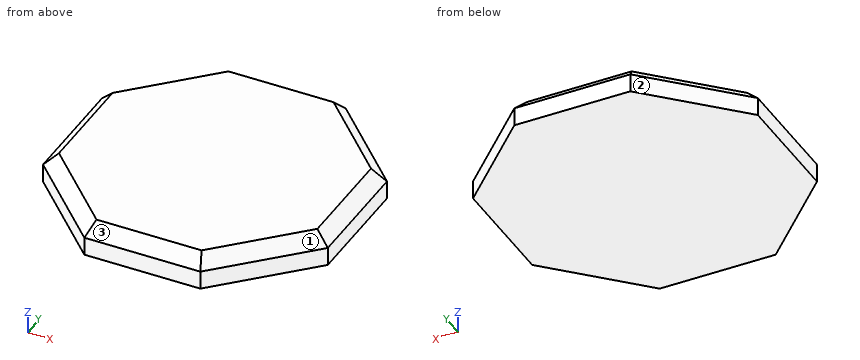
```python
from build123d import *

# Parameters (mm, degrees)
F0_W      = 171.45
F0_H      = 171.45
F1_DEPTH  = 19.05
F3_DEPTH  = 127
F2_W      = 12.7
F2_H      = 17.1814748066
F4_DEPTH  = 203.2
F5_SIZE   = 5.08
F6_DEPTH  = 177.8
F7_SIZE   = 5.08
F8_DEPTH  = 177.8
F9_SIZE   = 5.08
F2_H_2    = 15.875
F10_DEPTH = 152.4
F11_SIZE  = 5.08
F12_SIZE  = 50.8
F13_SIZE  = 7.9375
F15_R     = 19.8103080262
F16_DEPTH = 355.6
F17_SIZE  = 5.08
F18_DEPTH = 25.4


with BuildPart() as f1:
    # F0 (on Top) → F1 (new body)
    with BuildSketch(Plane.XY):
        Rectangle(F0_W, F0_H)
    extrude(amount=F1_DEPTH)

    # F12
    f12_edges = [f1.edges().sort_by_distance(p)[0] for p in [
        (85.725, 85.725, 9.525),
        (-85.725, 85.725, 9.525),
        (85.725, -85.725, 9.525),
        (-85.725, -85.725, 9.525),
    ]]
    chamfer(f12_edges, length=F12_SIZE)

    # F13
    f13_edges = [f1.edges().sort_by_distance(p)[0] for p in [
        (-60.325, -60.325, 19.05),
        (0, -85.725, 19.05),
        (60.325, -60.325, 19.05),
        (85.725, 0, 19.05),
        (60.325, 60.325, 19.05),
        (0, 85.725, 19.05),
        (-60.325, 60.325, 19.05),
        (-85.725, 0, 19.05),
    ]]
    chamfer(f13_edges, length=F13_SIZE)


with BuildPart() as f3:
    # F2 (on face) → F3 (new body)
    with BuildSketch(Plane.XY.offset(19.05)):
        Polygon((-8.0955186849, -20.6375), (7.9502, -20.6375), (20.6375, -9.2439748066), (20.6375, 7.9375), (7.9502, 20.6375), (-7.8052744357, 20.6375), (-20.6375, 7.9375), (-20.6375, -7.9375), align=None)
    extrude(amount=F3_DEPTH)


with BuildPart() as f4:
    # F2 (on face) → F4 (new body)
    with BuildSketch(Plane.XY.offset(19.05)):
        with Locations((26.9875, -0.6532374033)):
            Rectangle(F2_W, F2_H)
    extrude(amount=F4_DEPTH)

    # F5
    f5_edges = [f4.edges().sort_by_distance(p)[0] for p in [
        (33.3375, -0.653237, 222.25),
    ]]
    chamfer(f5_edges, length=F5_SIZE)


with BuildPart() as f6:
    # F2 (on face) → F6 (new body)
    with BuildSketch(Plane.XY.offset(19.05)):
        Polygon((-8.1848246077, -33.3375), (7.9502, -33.3375), (7.9502, -20.6375), (-8.0955186849, -20.6375), align=None)
    extrude(amount=F6_DEPTH)

    # F7
    f7_edges = [f6.edges().sort_by_distance(p)[0] for p in [
        (-0.117312, -33.3375, 196.85),
    ]]
    chamfer(f7_edges, length=F7_SIZE)


with BuildPart() as f8:
    # F2 (on face) → F8 (new body)
    with BuildSketch(Plane.XY.offset(19.05)):
        Polygon((-7.8052744357, 20.6375), (7.9502, 20.6375), (7.9502, 33.3375), (-7.7159685129, 33.3375), align=None)
    extrude(amount=F8_DEPTH)

    # F9
    f9_edges = [f8.edges().sort_by_distance(p)[0] for p in [
        (0.117116, 33.3375, 196.85),
    ]]
    chamfer(f9_edges, length=F9_SIZE)


with BuildPart() as f10:
    # F2 (on face) → F10 (new body)
    with BuildSketch(Plane.XY.offset(19.05)):
        with Locations((-26.9875, 0)):
            Rectangle(F2_W, F2_H_2)
    extrude(amount=F10_DEPTH)

    # F11
    f11_edges = [f10.edges().sort_by_distance(p)[0] for p in [
        (-33.3375, 0, 171.45),
    ]]
    chamfer(f11_edges, length=F11_SIZE)


with BuildPart() as f16:
    # F15 (on face) → F16 (new body)
    with BuildSketch(Plane.XY.offset(146.05)):
        Circle(F15_R)
    extrude(amount=F16_DEPTH)

    # F17
    f17_edges = [f16.edges().sort_by_distance(p)[0] for p in [
        (-19.810308, 0, 501.65),
    ]]
    chamfer(f17_edges, length=F17_SIZE)


with BuildPart() as f18:
    # F14 (on face) → F18 (new body)
    with BuildSketch(Plane.XY.offset(146.05)):
        with BuildLine():
            Line((20.6375, -0.9718922405), (20.6375, 0.9718922405))
            ThreePointArc((20.6375, 0.9718922405), (19.6667538049, 6.3300691588), (17.3298010521, 11.2485099579))
            Line((17.3298010521, 11.2485099579), (11.2658427939, 17.3185382443))
            ThreePointArc((11.2658427939, 17.3185382443), (6.3399066616, 19.6635847266), (0.9718922405, 20.6375))
            Line((0.9718922405, 20.6375), (-0.9718922405, 20.6375))
            ThreePointArc((-0.9718922405, 20.6375), (-6.1694748401, 19.7177220027), (-10.9643715831, 17.5109547588))
            Line((-10.9643715831, 17.5109547588), (-17.3964546014, 11.1451490829))
            ThreePointArc((-17.3964546014, 11.1451490829), (-19.685507724, 6.2715043193), (-20.6375, 0.9718922405))
            Line((-20.6375, 0.9718922405), (-20.6375, -0.9718922405))
            ThreePointArc((-20.6375, -0.9718922405), (-19.6458745255, -6.3945754282), (-17.2555997462, -11.3620094251))
            Line((-17.2555997462, -11.3620094251), (-11.5771558663, -17.1119970437))
            ThreePointArc((-11.5771558663, -17.1119970437), (-6.5174339176, -19.6054593393), (-0.9718922405, -20.6375))
            Line((-0.9718922405, -20.6375), (0.9718922405, -20.6375))
            ThreePointArc((0.9718922405, -20.6375), (14.6090893073, -14.6090893073), (20.6375, -0.9718922405))
        make_face()
    extrude(amount=F18_DEPTH)


solid = f1.part
```
CAD build for the part. Positions are in the model's coordinates, mm. Face numbers are marked on the shaded views. Round coordinates to 2 decimals unless told otherwise and drop trailing zeros. Write each loop counter-clockwise with the first axis right and the second up, starting at its lowest first coordinate (ties: lowest second). Pieces come first, ordered by that corner, then holes. Notation, with made-up numbers: (77.25, 55.5) - (87.25, 55.5) arc R26 cw to (87.25, 92.5) - close; hole circle Ø8 at (24, 22). An arc over 180 degrees is marked (long way). Write item = value, one per line. Start each with the question number.
Q1. Mould opens along X. For the marked faces 1, 2 and 3 say: pulls with the +X half, pulls with the -X half, needs draft (parallel to the pull), parting line crosses it, or undercut.
Q2. Drop flat-ended pins along their axis: pin 1 (6 mm diameter, centred on x = -62.5, y = -16.5, fed in from -Z); pin 2 (3 mm diameter, centred on y = -20.5, z = 17, fed in from +X); pin 3 (2 mm diameter, centred on x = 58.5, z = 14, fed in from -Y); pin 4 (1 mm diameter, centred on x = 20.5, z = 13.5, fed in from -Y). Give the stop position or say it passes through.
Q3. Probe L1, parallel to Y at x = -76.5, z = 12.75; L2, parallel to X at y = -54, z = 3.75; L3, parallel to Z at x = -70, y = 44.5. List the from-to ranges inside material, lowest first. Write a range as from..to.
Q4. Band-saw the part on D-D (z = 16). Give the cut face in (x, y).
Q5. Band-saw the part on B-B (z = 5.5). Give the cut face in (x, y) (3 decimals).
Answers below:
q1.face_1 = pulls with the +X half
q1.face_2 = pulls with the -X half
q1.face_3 = needs draft
q2.pin_1 = 0
q2.pin_2 = 81.34
q2.pin_3 = -59.8
q2.pin_4 = -83.84
q3.L1 = -41.83..41.83
q3.L2 = -66.65..66.65
q3.L3 = 0..15.46
q4.outline = (-80.84, -32.9) - (-32.9, -80.84) - (32.9, -80.84) - (80.84, -32.9) - (80.84, 32.9) - (32.9, 80.84) - (-32.9, 80.84) - (-80.84, 32.9) - close
q5.outline = (-85.725, -34.925) - (-34.925, -85.725) - (34.925, -85.725) - (85.725, -34.925) - (85.725, 34.925) - (34.925, 85.725) - (-34.925, 85.725) - (-85.725, 34.925) - close
